Design review of the part built by this model. Coordinates are the model's own, in mm. Coordinates: 2 decimals unless noted, no trailing zeros. Loops run counter-clockwise (first coordinate to the right, second up) from the corner with the lowest first, then second, coordinate; pieces in that order, holes last. Notation, with made-up numbers: (26, 20.5) -> (77, 20.5) arc R7 cw to (77, 29.5) -> close; hole circle Ø7 at (72, 32.5). An arc over 180 degrees is marked (long way). Use one line per item in the form item = value. Start each with the question number.
1. Consider section A-A (y = 30.5). State the section outline as (x, z) points, then the cut area to 4 significant figures.
2. Consider section C-C (z = 95.5). State the section outline as (x, y) points.
3. For pin 1 (3 mm diameter, centred on x = 2.5, z = 114, fed in from +Y), flat-tipped, find the tip position at first contact; note if it passes through.
4. Consider section B-B (x = 2.25). State how many separate pieces and enclosed holes the cut face has, then the cut area to 3 significant figures.
5. Consider section D-D (y = 107.5). State the section outline as (x, z) points.
6. Wall thickness on line 1 (Y direction, x = 1.75, z = -94.5); line 2 (Z direction, x = 1, y = -21.5); line 3 (Z direction, x = 4.25, y = 35): over which ranges is each line inside the solid? List them lowest first. Write a range as from..to.
from build123d import *

# Parameters (mm, degrees)
SALIENTE_EXTRUIR1_DEPTH = 6.35
CROQUIS2_W              = 6.35
CROQUIS2_H              = 20
CORTAR_EXTRUIR1_DEPTH   = 10
CROQUIS3_W              = 6.35
CROQUIS3_H              = 286.16
SALIENTE_EXTRUIR2_DEPTH = 6.35
CROQUIS4_W              = 6.35
CROQUIS4_H              = 20
CORTAR_EXTRUIR2_DEPTH   = 6.35
CROQUIS5_W              = 20
CROQUIS5_H              = 6.35
CORTAR_EXTRUIR3_DEPTH   = 10
CROQUIS6_W              = 10
CROQUIS6_H              = 286.16
CROQUIS6_H_2            = 170
SALIENTE_EXTRUIR3_DEPTH = 6.35


with BuildPart() as part:
    # Croquis1 → Saliente-Extruir1 (new body)
    with BuildSketch(Plane(origin=(0, 0, 0), x_dir=(0, 0, -1), z_dir=(1, 0, 0))):
        Polygon((-117.242954184, -155.20246182), (-117.242954184, 14.79753818), (-47.242954184, 14.79753818), (-47.242954184, 70.95753818), (22.757045816, 70.95753818), (22.757045816, 130.95753818), (92.757045816, 130.95753818), (92.757045816, -155.20246182), align=None)
    extrude(amount=SALIENTE_EXTRUIR1_DEPTH)

    # Croquis2 → Cortar-Extruir1 (cut)
    with BuildSketch(Plane.ZY):
        with Locations((114.067954184, -27.20246182)):
            Rectangle(CROQUIS2_W, CROQUIS2_H)
        with Locations((114.067954184, -113.20246182)):
            Rectangle(CROQUIS2_W, CROQUIS2_H)
        with Locations((44.067954184, -25.20246182)):
            Rectangle(CROQUIS2_W, CROQUIS2_H)
        with Locations((44.067954184, -95.20246182)):
            Rectangle(CROQUIS2_W, CROQUIS2_H)
        with Locations((-25.932045816, 34.79753818)):
            Rectangle(CROQUIS2_W, CROQUIS2_H)
        with Locations((-25.932045816, -35.20246182)):
            Rectangle(CROQUIS2_W, CROQUIS2_H)
    extrude(amount=-CORTAR_EXTRUIR1_DEPTH, mode=Mode.SUBTRACT)

    # Croquis3 → Saliente-Extruir2 (add)
    with BuildSketch(Plane(origin=(0, 0, 0), x_dir=(0, 0, -1), z_dir=(1, 0, 0))):
        with Locations((95.932045816, -12.12246182)):
            Rectangle(CROQUIS3_W, CROQUIS3_H)
    extrude(amount=SALIENTE_EXTRUIR2_DEPTH)

    # Croquis4 → Cortar-Extruir2 (cut)
    with BuildSketch(Plane.ZY):
        with Locations((-95.932045816, -10.20246182)):
            Rectangle(CROQUIS4_W, CROQUIS4_H)
        with Locations((-95.932045816, 62.29753818)):
            Rectangle(CROQUIS4_W, CROQUIS4_H)
        with Locations((-95.932045816, -82.70246182)):
            Rectangle(CROQUIS4_W, CROQUIS4_H)
    extrude(amount=-CORTAR_EXTRUIR2_DEPTH, mode=Mode.SUBTRACT)

    # Croquis5 → Cortar-Extruir3 (cut)
    with BuildSketch(Plane(origin=(6.35, 0, 0), x_dir=(0, 0, -1), z_dir=(1, 0, 0))):
        with Locations((-79.062954184, -123.86746182)):
            Rectangle(CROQUIS5_W, CROQUIS5_H)
        with Locations((-9.062954184, -63.86746182)):
            Rectangle(CROQUIS5_W, CROQUIS5_H)
        with Locations((60.937045816, -3.86746182)):
            Rectangle(CROQUIS5_W, CROQUIS5_H)
    extrude(amount=-CORTAR_EXTRUIR3_DEPTH, mode=Mode.SUBTRACT)

    # Croquis6 → Saliente-Extruir3 (add)
    with BuildSketch(Plane(origin=(0, 0, 0), x_dir=(0, 0, -1), z_dir=(1, 0, 0))):
        with Locations((104.107045816, -12.12246182)):
            Rectangle(CROQUIS6_W, CROQUIS6_H)
        with Locations((-122.242954184, -70.20246182)):
            Rectangle(CROQUIS6_W, CROQUIS6_H_2)
    extrude(amount=SALIENTE_EXTRUIR3_DEPTH)


solid = part.part
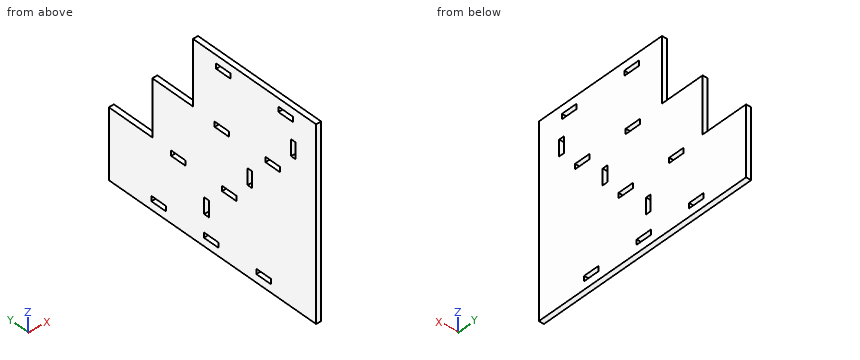
Geometry check:
q1.outline = (0, -109.11) -> (6.35, -109.11) -> (6.35, -29.11) -> (0, -29.11) -> close; (0, -22.76) -> (6.35, -22.76) -> (6.35, 47.24) -> (0, 47.24) -> close
q1.area = 952.5 mm²
q2.outline = (0, -155.2) -> (6.35, -155.2) -> (6.35, 14.8) -> (0, 14.8) -> close
q3.pin_1 = 14.8
q4.separate_pieces = 1
q4.enclosed_holes = 12
q4.area = 52,600 mm²
q5.outline = (0, -109.11) -> (6.35, -109.11) -> (6.35, -22.76) -> (0, -22.76) -> close
q6.line_1 = -155.2..-92.7, -72.7..-20.2, -0.2..52.3, 72.3..130.96
q6.line_2 = -109.11..40.89, 47.24..110.89, 117.24..127.24
q6.line_3 = -109.11..-29.11, -22.76..47.24
